from build123d import *

# Parameters (mm, degrees)
BOSS_EXTRUDE1_DEPTH     = 400
SKETCH2_W               = 100
SKETCH2_H               = 121
SKETCH2_W_2             = 95.3
SKETCH2_H_2             = 9.4
CUT_EXTRUDE1_DEPTH      = 268
CUT_EXTRUDE2_DEPTH      = 1
CUT_EXTRUDE2_DEPTH_BACK = 1161.696902422


with BuildPart() as part:
    # Sketch1 → Boss-Extrude1 (new body)
    with BuildSketch(Plane(origin=(0, 0, 0), x_dir=(0, 0, -1), z_dir=(1, 0, 0))):
        Polygon((0, 0), (-340, 0), (-350, 10), (-350, 960), (-310, 1000), (-158.48888922, 1000), (-158.48888922, 1160.696902422), (-108.48888922, 1160.696902422), (0, 1160.696902422), (0, 1000), (0, 970), (0, 820), (-9.396926208, 806.579798567), (-27.474774195, 800), (-190.603073792, 740.62615458), (-200, 727.205953147), (-200, 5), (0, 5), align=None)
    extrude(amount=BOSS_EXTRUDE1_DEPTH)

    # Sketch2 → Cut-Extrude1 (cut)
    with BuildSketch(Plane.XY.offset(350)):
        with Locations((200, 889.5)):
            Rectangle(SKETCH2_W, SKETCH2_H)
        with Locations((325, 889.5)):
            Rectangle(SKETCH2_W_2, SKETCH2_H_2)
    extrude(amount=-CUT_EXTRUDE1_DEPTH, mode=Mode.SUBTRACT)

    # Sketch3 → Cut-Extrude2 (cut, two sides)
    with BuildSketch(Plane(origin=(0, 0, 0), x_dir=(-1, 0, 0), z_dir=(0, -1, 0))) as cut_extrude2_sk:
        Polygon((32.971910004, -72.804395349), (-67.728153305, 29.569560354), (-322.648629759, 29.569560354), (-423.348693067, -72.804395349), (-423.348693067, 100.069531779), (32.971910004, 100.069531779), align=None)
    extrude(amount=CUT_EXTRUDE2_DEPTH, mode=Mode.SUBTRACT)
    extrude(cut_extrude2_sk.sketch, amount=-CUT_EXTRUDE2_DEPTH_BACK, mode=Mode.SUBTRACT)


solid = part.part
Geometry check sheet. Reference: the model listing, model coordinates, mm. A direction names the side the tool comes from. Coordinates: 2 decimals unless noted, no trailing zeros. Order: outer loops, then holes, each group sorted by start corner. A loop starts at its lowest first (then second) coordinate and runs counter-clockwise, first axis right, second up. Notation, with made-up numbers: (-26, 59) -> (-21, 59) arc R17 cw to (-21, 65) -> close; hole circle Ø9 at (23.5, 76.5). An arc over 180 degrees is marked (long way). Use a Markdown table: item, result. Add a question column.
1. Cross-section at C-C (y = 914.5). Enter the section's corners in (x, z), and give its area (3 significant figures).
2. Set-up check for faces 1 (the face through (150, 889, 218)), 2 (the face through (197, 5, 101)), 3 (the face through (197, 1160.697, 78)), 4 (the face through (197, 1000, 235)), 5 (the face through (19.05, 2.46, 19.92)): record each of +Z, -Z, +X, -X, +Y, -Y from which the full face is reachable in a straight line by a thin tool's end or side.
3. Cross-section at D-D (x = 223.5). Enter the section's corners in (y, z).
4. Material ranges on L1, parallel to Y at x = 337.5, z = 220.5; L2, parallel to Y at x = 247.5, z = 161.5; L3, parallel to Y at x = 359, z = 109, recorded low to high.
5. Mould release check, pull along X, two halves, no side actions. Record for faces 6 (the face through (400, 588, 231)), 7 (the face through (324, 884.8, 218)), 8 (the face through (197, 371, 200)): pulls with the +X half, pulls with the -X half, needs draft (parallel to the pull), parting line crosses it, or undercut.
6. Cross-section at B-B (z = 122). Enter the section's corners in (x, y), and give its area (3 significant figures).
7. Go/stop test with flat-tipped pins: pin 1 Ø1.5 at (x, y) = (157, 424.5) entering from -Z; pin 2 Ø5 at (x, y) = (283, 731.5) entering from -Z; pin 3 Ø4.5 at (x, y) = (329.5, 889) entering from +Z. Record where each tip stops, or that it passes through.
8. Cross-section at A-A (z = 232). Enter the section's corners in (x, y).
Filled sheet:
| question | item | result |
|---|---|---|
| 1 | outline | (0, 39.28) -> (38.64, 0) -> (351.73, 0) -> (400, 49.07) -> (400, 350) -> (250, 350) -> (250, 82) -> (150, 82) -> (150, 350) -> (0, 350) -> close |
| 1 | area | 111,000 mm2 |
| 2 | face 1 | +Z |
| 2 | face 2 | -Z, +X, -X |
| 2 | face 3 | +Z, -Z, +X, -X, +Y |
| 2 | face 4 | +Z, +X, -X, +Y |
| 2 | face 5 | -Z, -X, +Y, -Y |
| 3 | outline | (0, 0) -> (5, 0) -> (5, 200) -> (727.21, 200) -> (740.63, 190.6) -> (806.58, 9.4) -> (820, 0) -> (1160.7, 0) -> (1160.7, 158.49) -> (1000, 158.49) -> (1000, 310) -> (960, 350) -> (950, 350) -> (950, 82) -> (829, 82) -> (829, 350) -> (10, 350) -> (0, 340) -> close |
| 4 | L1 | 0 to 884.8, 894.2 to 1000 |
| 4 | L2 | 0 to 5, 751.22 to 829, 950 to 1000 |
| 4 | L3 | 0 to 5, 770.33 to 884.8, 894.2 to 1160.7 |
| 5 | face 6 | pulls with the +X half |
| 5 | face 7 | undercut |
| 5 | face 8 | needs draft |
| 6 | outline | (0, 0) -> (400, 0) -> (400, 5) -> (0, 5) -> close; (0, 765.6) -> (400, 765.6) -> (400, 1160.7) -> (0, 1160.7) -> close; hole (150, 829) -> (250, 829) -> (250, 950) -> (150, 950) -> close; hole (277.35, 884.8) -> (372.65, 884.8) -> (372.65, 894.2) -> (277.35, 894.2) -> close |
| 6 | area | 147,000 mm2 |
| 7 | pin 1 | z = 200 |
| 7 | pin 2 | z = 195.24 |
| 7 | pin 3 | z = 82 |
| 8 | outline | (0, 0) -> (400, 0) -> (400, 1000) -> (0, 1000) -> close; hole (150, 829) -> (250, 829) -> (250, 950) -> (150, 950) -> close; hole (277.35, 884.8) -> (372.65, 884.8) -> (372.65, 894.2) -> (277.35, 894.2) -> close |
